```python
from build123d import *

# Parameters (mm, degrees)
ESQUISSE1_R             = 2
ESQUISSE1_W             = 5
ESQUISSE1_H             = 5
BOSS_EXTRU_1_DEPTH      = 5
CONG_1_R                = 5
ESQUISSE2_W             = 13
ESQUISSE2_H             = 10
ENL_V_MAT_EXTRU_1_DEPTH = 61.671245248
CONG_2_R                = 3


with BuildPart() as part:
    # Esquisse1 → Boss.-Extru.1 (new body)
    with BuildSketch(Plane.XY):
        Polygon((34, 50), (34, 18.634320993), (21, 18.634320993), (6.358747791, 0), (21, -18.634320993), (34, -18.634320993), (34, -50), (21, -50), (21, -34.820224461), (0, -8.092951734), (-21, -34.820224461), (-21, -50), (-34, -50), (-34, -18.634320993), (-21, -18.634320993), (-6.358747791, 0), (-21, 18.634320993), (-34, 18.634320993), (-34, 50), (-21, 50), (-21, 34.820224461), (0, 8.092951734), (21, 34.820224461), (21, 50), align=None)
        with Locations((27.5, 35)):
            Circle(ESQUISSE1_R, mode=Mode.SUBTRACT)
        with Locations(Location((-27.5, 35, 0), (0, 0, 180))):
            Circle(ESQUISSE1_R, mode=Mode.SUBTRACT)
        with Locations((-27.5, -35)):
            Circle(ESQUISSE1_R, mode=Mode.SUBTRACT)
        with Locations(Location((27.5, -35, 0), (0, 0, 90))):
            Circle(ESQUISSE1_R, mode=Mode.SUBTRACT)
        with Locations((27.5, 27.5)):
            Rectangle(ESQUISSE1_W, ESQUISSE1_H, mode=Mode.SUBTRACT)
        with Locations((27.5, 42.5)):
            Rectangle(ESQUISSE1_W, ESQUISSE1_H, mode=Mode.SUBTRACT)
        with Locations((-27.5, 27.5)):
            Rectangle(ESQUISSE1_W, ESQUISSE1_H, mode=Mode.SUBTRACT)
        with Locations((-27.5, 42.5)):
            Rectangle(ESQUISSE1_W, ESQUISSE1_H, mode=Mode.SUBTRACT)
        with Locations((-27.5, -27.5)):
            Rectangle(ESQUISSE1_W, ESQUISSE1_H, mode=Mode.SUBTRACT)
        with Locations((-27.5, -42.5)):
            Rectangle(ESQUISSE1_W, ESQUISSE1_H, mode=Mode.SUBTRACT)
        with Locations((27.5, -27.5)):
            Rectangle(ESQUISSE1_W, ESQUISSE1_H, mode=Mode.SUBTRACT)
        with Locations((27.5, -42.5)):
            Rectangle(ESQUISSE1_W, ESQUISSE1_H, mode=Mode.SUBTRACT)
    extrude(amount=BOSS_EXTRU_1_DEPTH)

    # Congé1
    cong_1_edges = [part.edges().sort_by_distance(p)[0] for p in [
        (34, 50, 2.5),
        (34, 18.634320993, 2.5),
        (21, 18.634320993, 2.5),
        (6.358747791, 0, 2.5),
        (21, -18.634320993, 2.5),
        (34, -18.634320993, 2.5),
        (34, -50, 2.5),
        (21, -50, 2.5),
        (21, -34.820224461, 2.5),
        (0, -8.092951734, 2.5),
        (-21, -34.820224461, 2.5),
        (-21, -50, 2.5),
        (-34, -50, 2.5),
        (-34, -18.634320993, 2.5),
        (-21, -18.634320993, 2.5),
        (-6.358747791, 0, 2.5),
        (-21, 18.634320993, 2.5),
        (-34, 18.634320993, 2.5),
        (-34, 50, 2.5),
        (-21, 50, 2.5),
        (-21, 34.820224461, 2.5),
        (0, 8.092951734, 2.5),
        (21, 34.820224461, 2.5),
        (21, 50, 2.5),
    ]]
    fillet(cong_1_edges, radius=CONG_1_R)

    # Esquisse2 → Enlèv. mat.-Extru.1 (cut, through all)
    with BuildSketch(Plane.XY.offset(5)):
        with Locations((-27.5, 45)):
            Rectangle(ESQUISSE2_W, ESQUISSE2_H)
    extrude(amount=-ENL_V_MAT_EXTRU_1_DEPTH, mode=Mode.SUBTRACT)

    # Congé2
    cong_2_edges = [part.edges().sort_by_distance(p)[0] for p in [
        (-21, 40, 2.5),
        (-34, 40, 2.5),
    ]]
    fillet(cong_2_edges, radius=CONG_2_R)


solid = part.part
```
Could you check a few things on this model? Use its own coordinates, in mm. A direction names the side the tool comes from. Round coordinates to 2 decimals unless told otherwise and drop trailing zeros. Loops run counter-clockwise (first coordinate to the right, second up) from the corner with the lowest first, then second, coordinate; pieces in that order, holes last.
Q1. For P1, Ø1, axis at x = -22, y = -30.5, coming from the -Z side; P2, Ø2.5, axis at x = -28.5, z = 3.5, coming from the +Y side; P3, Ø3, axis at x = 11.5, z = 3.5, coming from the +Y side; P4, Ø1, axis at y = 6.5, z = 4, coming from the -X side, each with a flat end and sliding along its axis, tell me the tip position at first contact or that it passes through.
Q2. I want a section at D-D (x = 12). Write out the boundary of the cut face in (y, z), and give its area (3 significant figures).
Q3. I want a section at A-A (x = 27.5). Give the number of separate pieces and of enclosed holes in the cut face, and give its area (3 significant figures).
Q4. I want a section at B-B (x = -27.5). Write out the boundary of the cut face in (y, z), and give its area (3 significant figures).
Q5. I want a section at C-C (y = 22.5). Write out the boundary of the cut face in (x, z), and give its area (3 significant figures).
Q6. Please list where these lines run through material, in increasing order: L1, parallel to X at y = 25.5, z = 1.7; L2, parallel to X at y = -26.5, z = 3.95; L3, parallel to X at y = -23, z = 1.25.
Q7. Thinking about a two-plate mould opening in Y: for faces 1 (the cylindrical face through (-28.423, 36.774, 2.465)), 2 (the cylindrical face through (20.733, -34.937, 2.535)), 3 (the flat face through (25, -28, 2)), 4 (the flat face through (34, -34, 2)), which applies, pulls with the +Y half, pulls with the -Y half, needs draft (parallel to the pull), parting line crosses it, or undercut?
Q8. On a 3-axis mill with a long thin cutter (end or side, diameter ignored), from which of +Z, -Z, +X, -X, +Y, -Y can I reach the whole of each face in a straight line? I mean faces 5 (the cylindrical face through (21.22, -18.12, 2.54)), 6 (the flat face through (-34, -34, 2)), 7 (the flat face through (0, 1, 0)), 8 (the flat face through (30, 42, 2)), 9 (the flat face through (12.044, -23.421, 2.465)). Say none if no direction works.
Answer below:
1. P1: stops at z = 0
1. P2: stops at y = 40
1. P3: stops at y = 24.64
1. P4: stops at x = -11.86
2. outline: (-23.37, 0) - (-7.18, 0) - (-7.18, 5) - (-23.37, 5) - close; (7.18, 0) - (23.37, 0) - (23.37, 5) - (7.18, 5) - close
2. area: 162 mm2
3. separate pieces: 8
3. enclosed holes: 0
3. area: 174 mm2
4. outline: (-50, 0) - (-45, 0) - (-45, 5) - (-50, 5) - close; (-40, 0) - (-37, 0) - (-37, 5) - (-40, 5) - close; (-33, 0) - (-30, 0) - (-30, 5) - (-33, 5) - close; (-25, 0) - (-18.63, 0) - (-18.63, 5) - (-25, 5) - close; (18.63, 0) - (25, 0) - (25, 5) - (18.63, 5) - close; (30, 0) - (33, 0) - (33, 5) - (30, 5) - close; (37, 0) - (40, 0) - (40, 5) - (37, 5) - close
4. area: 149 mm2
5. outline: (-33.87, 0) - (-11.32, 0) - (-11.32, 5) - (-33.87, 5) - close; (11.32, 0) - (33.87, 0) - (33.87, 5) - (11.32, 5) - close
5. area: 225 mm2
6. L1: x = -34 to -30, -25 to -13.68, 13.68 to 25, 30 to 34
6. L2: x = -34 to -30, -25 to -14.46, 14.46 to 25, 30 to 34
6. L3: x = -33.96 to -11.71, 11.71 to 33.96
7. face 1: undercut
7. face 2: pulls with the -Y half
7. face 3: undercut
7. face 4: needs draft
8. face 5: +Z, -Z, +X
8. face 6: +Z, -Z, -X, +Y, -Y
8. face 7: -Z, +X, -X, +Y, -Y
8. face 8: +Z, -Z
8. face 9: +Z, -Z, -Y
